```python
from build123d import *

# Parameters (mm, degrees)
BOSS_EXTRUDE1_DEPTH = 4
SKETCH2_W           = 5
SKETCH2_H           = 10
BOSS_EXTRUDE2_DEPTH = 10
CUT_EXTRUDE1_REACH  = 7
SKETCH3_R           = 1.55


with BuildPart() as part:
    # Sketch1 → Boss-Extrude1 (new body)
    with BuildSketch(Plane.XY):
        with BuildLine():
            Line((2.823656605, 9.868817417), (18.486372689, 14.688114674))
            ThreePointArc((18.486372689, 14.688114674), (26.042750669, 15.988011567), (33.681837484, 15.33003533))
            Line((33.681837484, 15.33003533), (67.274577866, 8.027265681))
            ThreePointArc((67.274577866, 8.027265681), (70.67158791, 5.929345796), (72, 2.164207498))
            Line((72, 2.164207498), (72, -2.164207498))
            ThreePointArc((72, -2.164207498), (70.67158791, -5.929345796), (67.274577866, -8.027265681))
            Line((67.274577866, -8.027265681), (33.681837484, -15.33003533))
            ThreePointArc((33.681837484, -15.33003533), (26.042750669, -15.988011567), (18.486372689, -14.688114674))
            Line((18.486372689, -14.688114674), (2.823656605, -9.868817417))
            ThreePointArc((2.823656605, -9.868817417), (0.782440864, -8.422109009), (0, -6.045701382))
            Line((0, -6.045701382), (0, 6.045701382))
            ThreePointArc((0, 6.045701382), (0.782440864, 8.422109009), (2.823656605, 9.868817417))
        make_face()
    extrude(amount=BOSS_EXTRUDE1_DEPTH)

    # Sketch2 → Boss-Extrude2 (add)
    with BuildSketch(Plane(origin=(0, 0, 0), x_dir=(-1, 0, 0), z_dir=(0, 0, -1))):
        with Locations((-2.5, 0)):
            Rectangle(SKETCH2_W, SKETCH2_H)
    extrude(amount=BOSS_EXTRUDE2_DEPTH)

    # Sketch3 → Cut-Extrude1 (cut, up to next)
    with BuildSketch(Plane(origin=(5, 0, 0), x_dir=(0, 0, -1), z_dir=(1, 0, 0)), mode=Mode.PRIVATE) as cut_extrude1_sk1:
        with Locations((5, 0)):
            Circle(SKETCH3_R)
    cut_extrude1_tool1 = extrude(cut_extrude1_sk1.sketch, amount=-CUT_EXTRUDE1_REACH, mode=Mode.PRIVATE) & part.part
    add(cut_extrude1_tool1.solids().sort_by_distance((5, 0, -5))[0], mode=Mode.SUBTRACT)


solid = part.part
```
The listing builds one solid part. Answer for the finished solid, in the listing's coordinates (mm). A direction names the side the tool comes from. Give positions to 0.01 mm unless a question says otherwise; leave off trailing zeros. Order: outer loops, then holes, each group sorted by start corner. A loop starts at its lowest first (then second) coordinate and runs counter-clockwise, first axis right, second up. Notation, with made-up numbers: M -17.5,76 L 24.5,76 A14 ccw 24.5,102 Z; hole C 61,73.25 d2. An arc over 180 degrees is marked long. Put each result on its own line as item: value. Start each with the question number.
Item 1: Find the intervals of material crossed by line 1 along Y through (x, z) = (1.4, -5); line 2 along Z through (x, y) = (31, 0.5); line 3 along X through (y, z) = (-4.5, -4), in increasing order.
Item 2: The part is cut by section D-D, the plane y = 4. Determine the outline of the cut face in (x, z), and give its area (3 significant figures).
Item 3: The part is cut by section A-A, the plane y = 0. Determine the outline of the cut face in (x, z), and give its area (4 significant figures).
Item 4: The part is cut by section C-C, the plane z = 1. Determine the outline of the cut face in (x, y), and give its area (3 significant figures).
Item 5: Which of the six approach directions +Z, -Z, +X, -X, +Y, -Y give full straight-line access (tool end or side, diameter ignored) to faces 1 (the face through (10.545, 12.245, 1.972)), 2 (the face through (3, 5, -5)), 3 (the face through (5, 0, -3))?
Item 6: Flat-ended cylindrical pins translate along their axes: P1, Ø3, axis at x = 44, y = 11, coming from the -Z side; P2, Ø4, axis at y = 0, z = -5, coming from the -X side; P3, Ø5.5, axis at x = 2.5, z = -3, coming from the -Y side; P4, Ø2.5, axis at x = 3, z = -5.5, coming from the +Y side. Find the tip coordinate at first contact, or state that the pin passes through.
Item 7: For a pull along Y with two mould halves and no side action, classify faces 4 (the face through (25.935, 15.983, 1.972)), 5 (the face through (2.54, 0.07, -3.45)), 6 (the face through (3, -5, -5)), 7 (the face through (72, 0, 2)) as +Y half, -Y half, draft (parallel to the pull), parting line (faces both ways), or undercut.
Item 8: The part is cut by section B-B, the plane z = -5. Determine the outline of the cut face in (x, y), and give its area (3 significant figures).
Answer key:
1. line 1: y = -5 to -1.55, 1.55 to 5
1. line 2: z = 0 to 4
1. line 3: x = 0 to 5
2. outline: M 0,-10 L 5,-10 L 5,0 L 71.71,0 L 71.71,4 L 0,4 Z
2. area: 337 mm²
3. outline: M 0,-10 L 5,-10 L 5,-6.55 L 0,-6.55 Z; M 0,-3.45 L 5,-3.45 L 5,0 L 72,0 L 72,4 L 0,4 Z
3. area: 322.5 mm²
4. outline: M 0,-6.05 A4 ccw 2.82,-9.87 L 18.49,-14.69 A30 ccw 33.68,-15.33 L 67.27,-8.03 A6 ccw 72,-2.16 L 72,2.16 A6 ccw 67.27,8.03 L 33.68,15.33 A30 ccw 18.49,14.69 L 2.82,9.87 A4 ccw 0,6.05 Z
4. area: 1,760 mm²
5. face 1: +Z, -Z, -X, +Y
5. face 2: -Z, +X, -X, +Y
5. face 3: -Z, +X, +Y, -Y
6. P1: stops at z = 0
6. P2: stops at x = 0
6. P3: stops at y = -5
6. P4: stops at y = 5
7. face 4: +Y half
7. face 5: undercut
7. face 6: -Y half
7. face 7: draft
8. outline: M 0,-5 L 5,-5 L 5,-1.55 L 0,-1.55 Z; M 0,1.55 L 5,1.55 L 5,5 L 0,5 Z
8. area: 34.5 mm²
